Autodesk Inventor part; units mm, degrees
ref_plane "YZ Plane" through (0, 0, 0) normal (1, 0, 0) x (0, 1, 0)
ref_plane "XZ Plane" through (0, 0, 0) normal (0, 1, 0) x (-1, 0, 0)
ref_plane "XY Plane" through (0, 0, 0) normal (0, 0, 1) x (1, 0, 0)
sketch "Sketch1" plane through (0, 0, 0) normal (0, 0, 1) x (1, 0, 0)
  line L0 (-18.7833, 39.6114) -> (-18.7833, -39.6114)
  line L1 (-18.7833, -39.6114) -> (18.7833, -39.6114)
  line L2 (18.7833, -39.6114) -> (18.7833, 39.6114)
  line L3 (18.7833, 39.6114) -> (-18.7833, 39.6114)
  line L4 (-15.6083, 36.4364) -> (15.6083, 36.4364)
  line L5 (15.6083, 36.4364) -> (15.6083, -36.4364)
  line L6 (15.6083, -36.4364) -> (-15.6083, -36.4364)
  line L7 (-15.6083, -36.4364) -> (-15.6083, 36.4364)
  point P0 (0, 0)
extrude "Extrusion1" add sketch "Sketch1" along normal blind 3.175 contours L3 L2 L1 L0 | L4 L5 L6 L7
sketch "Sketch2" plane through (0, 0, 0) normal (0, 0, -1) x (-1, 0, 0)
  line L0 (-15.6083, -36.4364) -> (15.6083, -36.4364)
  line L1 (-15.6083, 36.4364) -> (-15.6083, -36.4364)
  line L2 (15.6083, 36.4364) -> (-15.6083, 36.4364)
  line L3 (15.6083, -36.4364) -> (15.6083, 36.4364)
  line L4 (-15.3543, 36.1824) -> (-15.3543, -36.1824)
  line L5 (-15.3543, -36.1824) -> (15.3543, -36.1824)
  line L6 (15.3543, -36.1824) -> (15.3543, 36.1824)
  line L7 (15.3543, 36.1824) -> (-15.3543, 36.1824)
  point P0 (0, 0)
  dimension "d2" = 0.254
extrude "Extrusion2" add sketch "Sketch2" along normal blind 1.5875 contours L7 L6 L5 L4
sketch "Sketch3" plane through (0, 0, -1.5875) normal (0, 0, -1) x (-1, 0, 0)
  line L0 (-15.3543, 36.1824) -> (-15.3543, -36.1824)
  line L1 (-15.3543, 36.1824) -> (-9.0043, 36.1824)
  line L2 (-9.0043, 36.1824) -> (-9.0043, 29.8324)
  line L3 (-9.0043, 29.8324) -> (-15.3543, 29.8324)
  line L4 (-15.3543, 29.8324) -> (-15.3543, 36.1824)
  line L5 (15.3543, 36.1824) -> (-15.3543, 36.1824)
  line L6 (15.3543, 36.1824) -> (9.0043, 36.1824)
  line L7 (9.0043, 36.1824) -> (9.0043, 29.8324)
  line L8 (9.0043, 29.8324) -> (15.3543, 29.8324)
  line L9 (15.3543, 29.8324) -> (15.3543, 36.1824)
  line L10 (-15.3543, -36.1824) -> (15.3543, -36.1824)
  line L11 (-15.3543, -36.1824) -> (-9.0043, -36.1824)
  line L12 (-9.0043, -36.1824) -> (-9.0043, -29.8324)
  line L13 (-9.0043, -29.8324) -> (-15.3543, -29.8324)
  line L14 (-15.3543, -29.8324) -> (-15.3543, -36.1824)
  line L15 (15.3543, 36.1824) -> (15.3543, -36.1824)
  line L16 (15.3543, -36.1824) -> (9.0043, -36.1824)
  line L17 (9.0043, -36.1824) -> (9.0043, -29.8324)
  line L18 (9.0043, -29.8324) -> (15.3543, -29.8324)
  line L19 (15.3543, -29.8324) -> (15.3543, -36.1824)
  point P0 (0, 0)
  dimension "d5" = 6.35
  dimension "d6" = 6.35
  dimension "d7" = 6.35
  dimension "d8" = 6.35
  dimension "d9" = 6.35
  dimension "d10" = 6.35
  dimension "d11" = 6.35
  dimension "d12" = 6.35
extrude "Extrusion3" add sketch "Sketch3" along normal blind 5.08 contours L1 L2 L3 L0 | L13 L12 L10 L0 | L5 L9 L8 L7 | L17 L18 L15 L10
sketch "Sketch4" plane through (15.3543, -36.1824, 0) normal (1, 0, 0) x (0, 0, -1)
  line L0 (6.6675, 66.0147) -> (6.6675, 72.3647)
  line L1 (0, 72.3647) -> (0, 0)
  line L2 (6.6675, 0) -> (6.6675, 6.35)
  line L3 (1.5875, 66.0147) -> (1.5875, 6.35)
  line L4 (0, 72.3647) -> (6.6675, 72.3647)
  line L5 (1.5875, 66.0147) -> (6.6675, 72.3647)
  line L6 (1.5875, 6.35) -> (6.6675, 6.35)
  line L7 (6.6675, 6.35) -> (6.6675, 0)
  line L8 (1.5875, 6.35) -> (6.6675, 0)
  point P0 (0, 36.1824)
  point P1 (4.1275, 3.175)
  point P2 (4.1275, 69.1897)
sketch "Sketch5" plane through (-15.3543, -36.1824, 0) normal (-1, 0, 0) x (0, 0, 1)
  point P0 (0, 36.1824)
  point P1 (-4.1275, 69.1897)
  point P2 (-4.1275, 3.175)
hole "Hole1" at (15.3543, 33.0074, -4.1275) at (15.3543, -33.0074, -4.1275) direction (-1, 0, 0) diameter 3.556 depth 5.842 countersink diameter 3.81 countersink angle 82
hole "Hole2" at (-15.3543, 33.0074, -4.1275) at (-15.3543, -33.0074, -4.1275) direction (1, 0, 0) diameter 3.556 depth 5.842 countersink diameter 3.81 countersink angle 82
sketch "Sketch6" plane through (0, 0, 3.175) normal (0, 0, 1) x (1, 0, 0)
  line L0 (-8.6233, 0) -> (8.6233, 0) construction
  line L1 (-8.6233, 2.54) -> (8.6233, 2.54)
  line L2 (8.6233, -2.54) -> (-8.6233, -2.54)
  arc A0 (-8.6233, 2.54) -> (-8.6233, -2.54) centre (-8.6233, 0) ccw
  arc A1 (8.6233, -2.54) -> (8.6233, 2.54) centre (8.6233, 0) ccw
  line L3 (-18.7833, 39.6114) -> (-18.7833, -39.6114)
  line L4 (18.7833, -39.6114) -> (18.7833, 39.6114)
  line L5 (-18.7833, -39.6114) -> (18.7833, -39.6114)
  arc A2 (8.6233, 10.16) -> (8.6233, 15.24) centre (8.6233, 12.7) ccw
  line L6 (-8.6233, 15.24) -> (8.6233, 15.24)
  line L7 (8.6233, 10.16) -> (-8.6233, 10.16)
  arc A3 (-8.6233, 15.24) -> (-8.6233, 10.16) centre (-8.6233, 12.7) ccw
  arc A4 (8.6233, 22.86) -> (8.6233, 27.94) centre (8.6233, 25.4) ccw
  line L8 (-8.6233, 27.94) -> (8.6233, 27.94)
  line L9 (8.6233, 22.86) -> (-8.6233, 22.86)
  arc A5 (-8.6233, 27.94) -> (-8.6233, 22.86) centre (-8.6233, 25.4) ccw
  arc A6 (8.6233, -15.24) -> (8.6233, -10.16) centre (8.6233, -12.7) ccw
  line L10 (-8.6233, -10.16) -> (8.6233, -10.16)
  line L11 (8.6233, -15.24) -> (-8.6233, -15.24)
  arc A7 (-8.6233, -10.16) -> (-8.6233, -15.24) centre (-8.6233, -12.7) ccw
  arc A8 (8.6233, -2.54) -> (8.6233, 2.54) centre (8.6233, 0) ccw
  line L12 (-8.6233, 2.54) -> (8.6233, 2.54)
  line L13 (8.6233, -2.54) -> (-8.6233, -2.54)
  arc A9 (-8.6233, 2.54) -> (-8.6233, -2.54) centre (-8.6233, 0) ccw
  arc A10 (8.6233, 10.16) -> (8.6233, 15.24) centre (8.6233, 12.7) ccw
  line L14 (-8.6233, 15.24) -> (8.6233, 15.24)
  line L15 (8.6233, 10.16) -> (-8.6233, 10.16)
  arc A11 (-8.6233, 15.24) -> (-8.6233, 10.16) centre (-8.6233, 12.7) ccw
  arc A12 (8.6233, -27.94) -> (8.6233, -22.86) centre (8.6233, -25.4) ccw
  line L16 (-8.6233, -22.86) -> (8.6233, -22.86)
  line L17 (8.6233, -27.94) -> (-8.6233, -27.94)
  arc A13 (-8.6233, -22.86) -> (-8.6233, -27.94) centre (-8.6233, -25.4) ccw
  arc A14 (8.6233, -15.24) -> (8.6233, -10.16) centre (8.6233, -12.7) ccw
  line L18 (-8.6233, -10.16) -> (8.6233, -10.16)
  line L19 (8.6233, -15.24) -> (-8.6233, -15.24)
  arc A15 (-8.6233, -10.16) -> (-8.6233, -15.24) centre (-8.6233, -12.7) ccw
  arc A16 (8.6233, -2.54) -> (8.6233, 2.54) centre (8.6233, 0) ccw
  line L20 (-8.6233, 2.54) -> (8.6233, 2.54)
  line L21 (8.6233, -2.54) -> (-8.6233, -2.54)
  arc A17 (-8.6233, 2.54) -> (-8.6233, -2.54) centre (-8.6233, 0) ccw
  point P0 (0, 0)
  point P1 (0, 0)
  dimension "d29" = 10.16
  dimension "d30" = 10.16
  dimension "d31" = 2.54
  dimension "d35" = 12.7
  dimension "d38" = 12.7
extrude "Extrusion4" cut sketch "Sketch6" against normal up to surface (4.7625 mm away)
properties part number "SENSOR_TOP" material "PC/ABS Plastic"
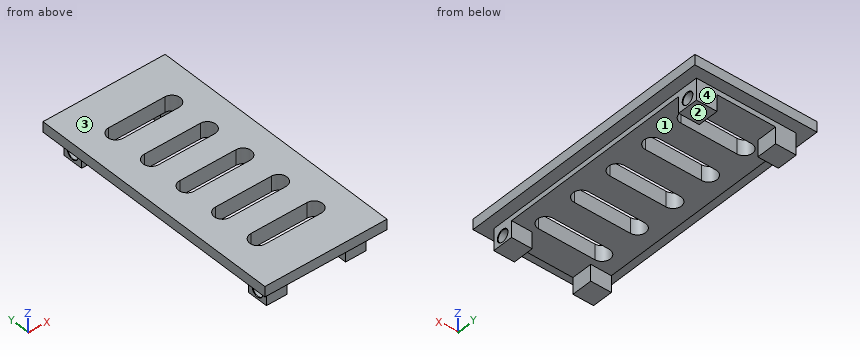
Verification items for the finished model (mm, model axes). Face numbers are marked on the shaded views. A direction names the side the tool comes from. Give positions to 0.01 mm unless a question says otherwise; leave off trailing zeros. Order: outer loops, then holes, each group sorted by start corner. A loop starts at its lowest first (then second) coordinate and runs counter-clockwise, first axis right, second up. Notation, with made-up numbers: M 29.5,74 L 60.5,74 A6 cw 60.5,85 Z; hole C -18.5,72 d2. An arc over 180 degrees is marked long. Answer as a JSON object with one key per item and string values. Group by question number.
1) Scan lines: line 1 along X through (y, z) = (32.5, -6); line 2 along Y through (x, z) = (7, 1.75); line 3 along X through (y, z) = (-13, -0.25). Record each from-to range of solid material in increasing order. Write a range as [from, to].
2) Cross-section at A-A (x = 6.5). Enter the section's corners in (y, z) (1 decimal).
3) Access from +Z, -Z, +X, -X, +Y, -Y to the whole of each face (thin tool, end or side, straight path). Record for the marked faces 3 and 4.
4) Depth check by flat-ended pin: pin 1 Ø1.8 at (y, z) = (33.5, -4.5) entering from -X; pin 2 Ø1.5 at (y, z) = (-33, -3.5) entering from +X; pin 3 Ø5 at (x, z) = (-8, -3.5) entering from +Y. Enter the tip coordinate at first touch or a pass-through.
5) Cross-section at B-B (y = 12.7). Enter the section's corners in (x, z) (1 decimal).
6) Mould release check, pull along X, two halves, no side actions. Record for the marked faces 1 and 2: released by +X, released by -X, zero draft, split by the parting line, or undercut.
7) Cross-section at D-D (z = -4). Give the number of separate pieces and of enclosed holes in the cut face, then the cut area to 3 significant figures.
Result sheet:
{
 "1": {"line 1": "x = [-15.35, -9], [9, 15.35]", "line 2": "y = [-39.61, -27.94], [-22.86, -15.24], [-10.16, -2.54], [2.54, 10.16], [15.24, 22.86], [27.94, 39.61]", "line 3": "x = [-15.35, -11.15], [11.15, 15.35]"},
 "2": {"outline": "M -39.6,0 L -36.2,0 L -36.2,-1.6 L -27.9,-1.6 L -27.9,3.2 L -39.6,3.2 Z; M -22.9,-1.6 L -15.2,-1.6 L -15.2,3.2 L -22.9,3.2 Z; M -10.2,-1.6 L -2.5,-1.6 L -2.5,3.2 L -10.2,3.2 Z; M 2.5,-1.6 L 10.2,-1.6 L 10.2,3.2 L 2.5,3.2 Z; M 15.2,-1.6 L 22.9,-1.6 L 22.9,3.2 L 15.2,3.2 Z; M 27.9,-1.6 L 36.2,-1.6 L 36.2,0 L 39.6,0 L 39.6,3.2 L 27.9,3.2 Z"},
 "3": {"face 3": "+Z, +X, -X, +Y, -Y", "face 4": "-Z, +X, -X, +Y"},
 "4": {"pin 1": "stops at x = -9.51", "pin 2": "stops at x = 9.51", "pin 3": "stops at y = 36.18"},
 "5": {"outline": "M -18.8,0 L -15.4,0 L -15.4,-1.6 L -11.2,-1.6 L -11.2,3.2 L -18.8,3.2 Z; M 11.2,-1.6 L 15.4,-1.6 L 15.4,0 L 18.8,0 L 18.8,3.2 L 11.2,3.2 Z"},
 "6": {"face 1": "undercut", "face 2": "zero draft"},
 "7": {"separate pieces": "4", "enclosed holes": "0", "area": "78.3 mm2"}
}
